Part model, mm, in its own coordinate system. Face numbers are marked on the shaded views. A direction names the side the tool comes from. Give positions to 0.01 mm unless a question says otherwise; leave off trailing zeros. Write each loop counter-clockwise with the first axis right and the second up, starting at its lowest first coordinate (ties: lowest second). Pieces come first, ordered by that corner, then holes. Notation, with made-up numbers: M 5,41 L 46,41 A23 cw 46,71 Z; hole C -24,48.25 d6. An arc over 180 degrees is marked long. Use CSV: the item, a comma, the result in double quotes. Start each with the question number.
1. Band-saw the part on D-D, the plane x = -17.5. List the corners of the cut face in (y, z).
2. 3-axis set-ups, long thin cutter, end or side, ignore diameter. For the marked faces 1 and 2: which of +Z, -Z, +X, -X, +Y, -Y reach the whole face in a straight line?
3. Drop flat-ended pins along their axis: pin 1 Ø1 at (y, z) = (4, 3.5) entering from +X; pin 2 Ø1 at (x, z) = (21, 1) entering from +Y; pin 3 Ø2 at (y, z) = (21.5, 1) entering from -X; pin 4 Ø3 at (x, y) = (7.5, 12) entering from -Z. Give the stop position or say it passes through.
4. Band-saw the part on C-C, the plane z = 6. List the corners of the cut face in (x, y).
5. Drill centre lines: line 1 along Z through (x, y) = (-2.5, 15); line 2 along Y through (x, z) = (-1, 7.75); line 3 along X through (y, z) = (6, 1). Where is each one in solid material? Low to high. Write a range as from..to.
6. Band-saw the part on A-A, the plane y = 0. List the corners of the cut face in (x, z), then the cut area to 3 significant figures.
from build123d import *

# Parameters (mm, degrees)
BOX_W          = 14
BOX_H          = 48
BOX_DEPTH      = 2
FILLET_R       = 1.5
BOX001_W       = 48
BOX001_H       = 14
BOX001_DEPTH   = 2
FILLET001_R    = 1.5
CYLINDER_R     = 21.5
CYLINDER_DEPTH = 2


with BuildPart() as cone:
    # Cone → Cone (revolve)
    with BuildSketch(Plane(origin=(0, 0, 2), x_dir=(1, 0, 0), z_dir=(0, -1, 0))):
        Polygon((0, 0), (11, 0), (13, 8), (0, 8), align=None)
    revolve(axis=Axis((0, 0, 2), (0, 0, 1)))


with BuildPart() as fillet_body:
    # Box → Box (new body)
    with BuildSketch(Plane(origin=(-7, -24, 0), x_dir=(1, 0, 0), z_dir=(0, 0, 1))):
        with Locations((7, 24)):
            Rectangle(BOX_W, BOX_H)
    extrude(amount=BOX_DEPTH)

    # Fillet
    fillet_edges = [fillet_body.edges().sort_by_distance(p)[0] for p in [
        (-7, -24, 1),
        (-7, 24, 1),
        (7, -24, 1),
        (7, 24, 1),
    ]]
    fillet(fillet_edges, radius=FILLET_R)


with BuildPart() as fillet001:
    # Box001 → Box001 (new body)
    with BuildSketch(Plane(origin=(-24, -7, 0), x_dir=(1, 0, 0), z_dir=(0, 0, 1))):
        with Locations((24, 7)):
            Rectangle(BOX001_W, BOX001_H)
    extrude(amount=BOX001_DEPTH)

    # Fillet001
    fillet001_edges = [fillet001.edges().sort_by_distance(p)[0] for p in [
        (-24, -7, 1),
        (-24, 7, 1),
        (24, -7, 1),
        (24, 7, 1),
    ]]
    fillet(fillet001_edges, radius=FILLET001_R)


with BuildPart() as obj1:
    # Cylinder → Cylinder (new body)
    with BuildSketch(Plane.XY):
        Circle(CYLINDER_R)
    extrude(amount=CYLINDER_DEPTH)

    # Fusion: union Cone, Fillet body, Fillet001
    add(cone.part)
    add(fillet_body.part)
    add(fillet001.part)


solid = obj1.part
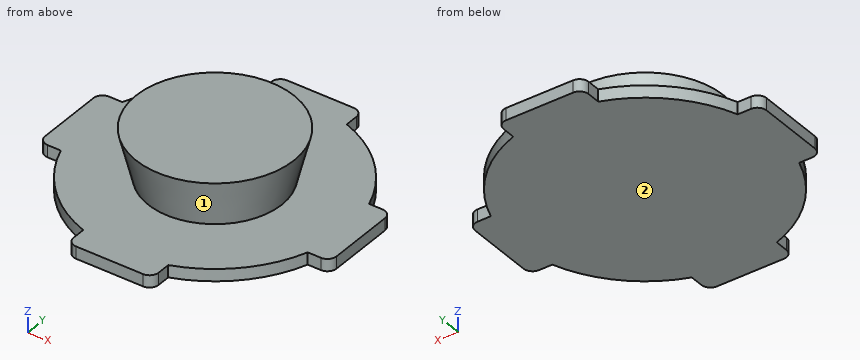
Output:
1,outline,"M -12.49,0 L 12.49,0 L 12.49,2 L -12.49,2 Z"
2,face 1,"none"
2,face 2,"-Z, +X, -X, +Y, -Y"
3,pin 1,"stops at x = 10.87"
3,pin 2,"stops at y = 7"
3,pin 3,"stops at x = -7"
3,pin 4,"stops at z = 0"
4,outline,"C 0,0 d24"
5,line 1,"z = 0..2"
5,line 2,"y = -12.4..12.4"
5,line 3,"x = -23.91..23.91"
6,outline,"M -24,0 L 24,0 L 24,2 L 11,2 L 13,10 L -13,10 L -11,2 L -24,2 Z"
6,area,"288 mm²"
